Here's how the part is built. I have some questions about the finished solid (model axes, mm). Coordinates: 2 decimals unless noted, no trailing zeros. Write each loop counter-clockwise with the first axis right and the second up, starting at its lowest first coordinate (ties: lowest second). Pieces come first, ordered by that corner, then holes. Notation, with made-up numbers: (17, 52) -> (30, 52) arc R22 cw to (30, 80) -> close; hole circle Ø1 at (0, 55). An arc over 180 degrees is marked (long way). Put each result on its own line as item: value. Start each with the question number.
Item 1: I want a section at B-B, the plane x = 17.5. List the corners of the cut face in (y, z) for me (3 decimals), then the cut area to 3 significant figures.
Item 2: I want a section at D-D, the plane y = -19.5. List the corners of the cut face in (x, z) for me (3 decimals).
Item 3: I need wall thicknesses on line 1 (Z direction, x = 12, y = 0); line 2 (Z direction, x = 10.5, y = 9); line 3 (Y direction, x = 20.25, z = 2). Which ranges of each line are inside material? Lowest first, please. Write a range as [from, to].
Item 4: I want a section at A-A, the plane z = 0. List the corners of the cut face in (x, y) for me.
Item 5: I want a section at C-C, the plane y = -1.5. List the corners of the cut face in (x, z) for me.
Item 6: For pin 1 (1.5 mm diameter, centred on y = 2, z = -14, fed in from -X); pin 2 (4 mm diameter, centred on x = 8.5, z = 7, fed in from +Y); pin 3 (10 mm diameter, centred on x = 9, z = 13.5, fed in from +Y), each with a flat end and sliding along its axis, tell me the tip position at first contact or that it passes through.
Item 7: If we mould it in two halves opening along Z, with no side actions, what happens to faces 1 (the face through (0, -7, -12)), 2 (the face through (12.522, 0.279, 19.048)), 3 (the face through (12.52, -2.75, -12.4)), 4 (the face through (12.522, -27.542, -15.794))? For each: released by +Z, released by -Z, zero draft, split by the parting line, or undercut.
from build123d import *

# Parameters (mm, degrees)
F0_R     = 12.7
F1_DEPTH = 25.4


with BuildPart() as f1:
    # F0 (on Right) → F1 (new body)
    with BuildSketch(Plane.YZ):
        with BuildLine():
            ThreePointArc((0, -19.05), (13.470384, -13.470384), (19.05, 0))
            ThreePointArc((19.05, 0), (18.400887, 4.930503), (16.497784, 9.525))
            ThreePointArc((16.497784, 9.525), (0, 19.05), (-16.497784, 9.525))
            ThreePointArc((-16.497784, 9.525), (-16.497784, -9.525), (0, -19.05))
        make_face()
        Circle(F0_R, mode=Mode.SUBTRACT)
        with BuildLine():
            ThreePointArc((16.497784, 9.525), (18.400887, 4.930503), (19.05, 0))
            ThreePointArc((19.05, 0), (13.470384, -13.470384), (0, -19.05))
            Line((0, -19.05), (21.997045, -19.05))
            ThreePointArc((21.997045, -19.05), (27.496307, -15.875), (27.496307, -9.525))
            Line((27.496307, -9.525), (16.497784, 9.525))
        make_face()
        with BuildLine():
            Line((-21.997045, -19.05), (0, -19.05))
            ThreePointArc((0, -19.05), (-16.497784, -9.525), (-16.497784, 9.525))
            Line((-16.497784, 9.525), (-27.496307, -9.525))
            ThreePointArc((-27.496307, -9.525), (-27.496307, -15.875), (-21.997045, -19.05))
        make_face()
    extrude(amount=F1_DEPTH)


solid = f1.part
Calculated:
1. outline: (-27.496, -9.525) arc R6.35 ccw to (-21.997, -19.05) -> (21.997, -19.05) arc R6.35 ccw to (27.496, -9.525) -> (16.498, 9.525) arc R19.05 ccw to (-16.498, 9.525) -> close; hole circle Ø25.4 at (0, 0)
1. area: 1,080 mm2
2. outline: (0, -19.05) -> (25.4, -19.05) -> (25.4, 4.325) -> (0, 4.325) -> close
3. line 1: z = [-19.05, -12.7], [12.7, 19.05]
3. line 2: z = [-19.05, -8.96], [8.96, 16.79]
3. line 3: y = [-20.84, -12.54], [12.54, 20.84]
4. outline: (0, -22) -> (25.4, -22) -> (25.4, -12.7) -> (0, -12.7) -> close; (0, 12.7) -> (25.4, 12.7) -> (25.4, 22) -> (0, 22) -> close
5. outline: (0, -19.05) -> (25.4, -19.05) -> (25.4, -12.61) -> (0, -12.61) -> close; (0, 12.61) -> (25.4, 12.61) -> (25.4, 18.99) -> (0, 18.99) -> close
6. pin 1: stops at x = 0
6. pin 2: stops at y = 19.11
6. pin 3: stops at y = 17.09
7. face 1: zero draft
7. face 2: released by +Z
7. face 3: undercut
7. face 4: split by the parting line
